```python
from build123d import *

# Parameters (mm, degrees)
F0_W     = 227.11908
F0_H     = 25.916077
F0_W_2   = 14.513008
F0_H_2   = 17.340212
F0_W_3   = 17.492868
F0_H_3   = 12.324523
F0_W_4   = 16.69774
F0_H_4   = 14.709914
F1_DEPTH = 25.4


with BuildPart() as f1:
    # F0 (on Front) → F1 (new body)
    with BuildSketch(Plane.XZ):
        with Locations((40.617559, 12.958038)):
            Rectangle(F0_W, F0_H)
        with Locations((-58.146257, 11.780035)):
            Rectangle(F0_W_2, F0_H_2, mode=Mode.SUBTRACT)
        with Locations((104.388017, 12.622695)):
            Rectangle(F0_W_3, F0_H_3, mode=Mode.SUBTRACT)
        with Locations((-2.358241, 15.008087)):
            Rectangle(F0_W_4, F0_H_4, mode=Mode.SUBTRACT)
    extrude(amount=F1_DEPTH)


solid = f1.part
```
Design review of the part built by this model. Coordinates are the model's own, in mm. A direction names the side the tool comes from. Round coordinates to 2 decimals unless told otherwise and drop trailing zeros. Write each loop counter-clockwise with the first axis right and the second up, starting at its lowest first coordinate (ties: lowest second). Pieces come first, ordered by that corner, then holes.
Item 1: We need section B-B on z = 14. Write out the cut boundary in (x, y), and give its area (3 significant figures).
Item 2: We need section A-A on x = 98. Write out the cut boundary in (y, z), and give its area (3 significant figures).
Item 3: The part is to be moulded in two halves that separate along X. For faces 1 (the flat face through (5.991, -13, 15)), 2 (the flat face through (154.177, -13, 13)), 3 (the flat face through (39, -13, 25.916)), say which applies: +X half, -X half, draft (parallel to the pull), parting line (faces both ways), or undercut.
Item 4: We need section D-D on x = -4. Write out the cut boundary in (y, z), and give its area (3 significant figures).
Item 5: For faces 4 (the flat face through (39, -25.4, 13)), 5 (the flat face through (-10.707, -13, 15)), list the 3-axis set-ups (+Z, -Z, +X, -X, +Y, -Y) from which the entire face can be reached by the end or side of a thin tool; tool diameter is ignored.
Item 6: We need section C-C on y = -9.75. Write out the cut boundary in (x, z), and give its area (3 significant figures).
Item 7: Clearance check with a flat-ended pin moving along its axis: pin 1 Ø6 at (x, z) = (-18, 6.5) entering from +Y. State where the tip first meets the part, or that it passes through.
Item 8: For probe 1 along X at (y, z) = (-23.5, 10.5); probe 2 along X at (y, z) = (-8.75, 21.25); probe 3 along Z at (x, y) = (106, -5), list the stretches that pass through material, from the lowest coordinate up.
Returned:
1. outline: (-72.94, -25.4) - (-65.4, -25.4) - (-65.4, 0) - (-72.94, 0) - close; (-50.89, -25.4) - (-10.71, -25.4) - (-10.71, 0) - (-50.89, 0) - close; (5.99, -25.4) - (95.64, -25.4) - (95.64, 0) - (5.99, 0) - close; (113.13, -25.4) - (154.18, -25.4) - (154.18, 0) - (113.13, 0) - close
1. area: 4,530 mm2
2. outline: (-25.4, 0) - (0, 0) - (0, 6.46) - (-25.4, 6.46) - close; (-25.4, 18.78) - (0, 18.78) - (0, 25.92) - (-25.4, 25.92) - close
2. area: 345 mm2
3. face 1: undercut
3. face 2: +X half
3. face 3: draft
4. outline: (-25.4, 0) - (0, 0) - (0, 7.65) - (-25.4, 7.65) - close; (-25.4, 22.36) - (0, 22.36) - (0, 25.92) - (-25.4, 25.92) - close
4. area: 285 mm2
5. face 4: +Z, -Z, +X, -X, -Y
5. face 5: +Y, -Y
6. outline: (-72.94, 0) - (154.18, 0) - (154.18, 25.92) - (-72.94, 25.92) - close; hole (-65.4, 3.11) - (-50.89, 3.11) - (-50.89, 20.45) - (-65.4, 20.45) - close; hole (-10.71, 7.65) - (5.99, 7.65) - (5.99, 22.36) - (-10.71, 22.36) - close; hole (95.64, 6.46) - (113.13, 6.46) - (113.13, 18.78) - (95.64, 18.78) - close
6. area: 5,170 mm2
7. pin 1: stops at y = 0
8. probe 1: x = -72.94 to -65.4, -50.89 to -10.71, 5.99 to 95.64, 113.13 to 154.18
8. probe 2: x = -72.94 to -10.71, 5.99 to 154.18
8. probe 3: z = 0 to 6.46, 18.78 to 25.92
